from build123d import *

# Parameters (mm, degrees)
SALIENTE_EXTRUIR1_DEPTH = 3.18


with BuildPart() as part:
    # Croquis1 → Saliente-Extruir1 (new body)
    with BuildSketch(Plane(origin=(0, 0, 0), x_dir=(1, 0, 0), z_dir=(0, 1, 0))):
        with BuildLine():
            Line((-4.765, 1.59418202), (4.765, 1.59418202))
            ThreePointArc((4.765, 1.59418202), (9.257217817, 2.411625687), (13.17, 4.765))
            Line((13.17, 4.765), (31.75, 4.765))
            Line((31.75, 4.765), (31.75, -4.765))
            Line((31.75, -4.765), (13.17, -4.765))
            ThreePointArc((13.17, -4.765), (9.258084222, -2.407173521), (4.765, -1.58581798))
            Line((4.765, -1.58581798), (-4.765, -1.58581798))
            ThreePointArc((-4.765, -1.58581798), (-9.258084222, -2.407173521), (-13.17, -4.765))
            Line((-13.17, -4.765), (-31.75, -4.765))
            Line((-31.75, -4.765), (-31.75, 4.765))
            Line((-31.75, 4.765), (-13.17, 4.765))
            ThreePointArc((-13.17, 4.765), (-9.257217817, 2.411625687), (-4.765, 1.59418202))
        make_face()
    extrude(amount=SALIENTE_EXTRUIR1_DEPTH)


solid = part.part
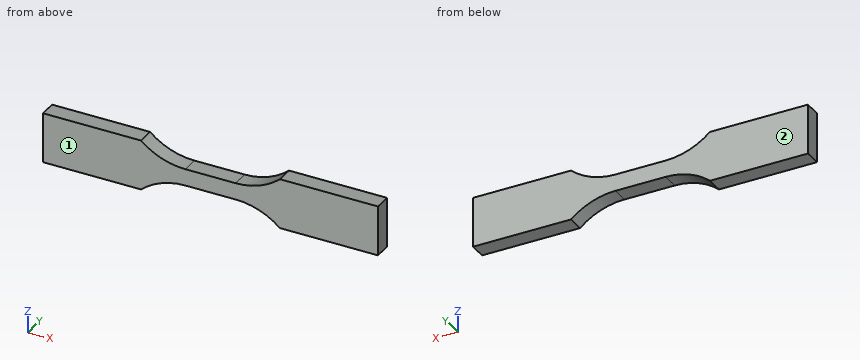
The listing builds one solid part. Answer for the finished solid, in the listing's coordinates (mm). Face numbers are marked on the shaded views. Round coordinates to 2 decimals unless told otherwise and drop trailing zeros. Order: outer loops, then holes, each group sorted by start corner. A loop starts at its lowest first (then second) coordinate and runs counter-clockwise, first axis right, second up. Notation, with made-up numbers: (54, 41) - (96, 41) arc R18 cw to (96, 68) - close; hole circle Ø6 at (-38, 12). An arc over 180 degrees is marked (long way). Write item = value, one per line. Start each with the question number.
1) Section A-A, the plane z = 3.25 is taken. Write down the section's boundary in (x, y), plus the area to 3 significant figures.
2) Section B-B, the plane y = 1.45 is taken. Write down the section's boundary in (x, z) (3 decimals).
3) Straight lines are drawn through the part: L1, parallel to Z at x = -1, y = 2.95; L2, parallel to X at y = 2.25, z = -2.5; L3, parallel to Z at x = -11, y = 2.55. For each, find the intervals that lie inside material, in ascending order.
4) Given pin 1 (1.6 mm diameter, centred on x = 2, y = 1, fed in from +Z), flat-ended and moving along its own axis, determine where the tip first touches the part or whether it passes through.
5) For a pull along Y with two mould halves and no side action, classify the marked faces 1 and 2 as released by +Y, released by -Y, zero draft, split by the parting line, or undercut.
6) Section D-D, the plane x = 11 is taken. Write down the section's boundary in (y, z), plus the area to 3 significant figures.
7) Section C-C, the plane z = -2.75 is taken. Write down the section's boundary in (x, y).
Results list:
q1.outline = (-31.75, 0) - (-11.05, 0) - (-11.05, 3.18) - (-31.75, 3.18) - close; (11.05, 0) - (31.75, 0) - (31.75, 3.18) - (11.05, 3.18) - close
q1.area = 132 mm^2
q2.outline = (-31.75, -4.765) - (-13.17, -4.765) arc R12.7 cw to (-4.765, -1.594) - (4.765, -1.594) arc R12.7 cw to (13.17, -4.765) - (31.75, -4.765) - (31.75, 4.765) - (13.17, 4.765) arc R12.7 cw to (4.765, 1.586) - (-4.765, 1.586) arc R12.7 cw to (-13.17, 4.765) - (-31.75, 4.765) - close
q3.L1 = -1.59 to 1.59
q3.L2 = -31.75 to -9.48, 9.48 to 31.75
q3.L3 = -3.22 to 3.22
q4.pin_1 = 1.59
q5.face_1 = released by -Y
q5.face_2 = released by +Y
q6.outline = (0, -3.22) - (3.18, -3.22) - (3.18, 3.22) - (0, 3.22) - close
q6.area = 20.5 mm^2
q7.outline = (-31.75, 0) - (-10.07, 0) - (-10.07, 3.18) - (-31.75, 3.18) - close; (10.07, 0) - (31.75, 0) - (31.75, 3.18) - (10.07, 3.18) - close
